from build123d import *

# Parameters (mm, degrees)
F1_DEPTH = 44
F2_R     = 2
F3_DEPTH = 25


with BuildPart() as f1:
    # F0 (on Front) → F1 (new body)
    with BuildSketch(Plane.XZ):
        Polygon((0, 2), (0, 0), (36, 0), (36, 2), (20, 2), (20, 14.713833), (36.245195, 32.134672), (50.505946, 32.134672), (50.505946, 36.134672), (34.505946, 36.134672), (12, 12), (12, 2), align=None)
    extrude(amount=-F1_DEPTH)

    # F2 (on Top) → F3 (cut)
    with BuildSketch(Plane.XY):
        with Locations((4, 40)):
            Circle(F2_R)
        with BuildLine():
            Line((12, 0), (12, 36))
            Line((12, 36), (4, 36))
            ThreePointArc((4, 36), (1.171573, 37.171573), (0, 40))
            Line((0, 40), (0, 0))
            Line((0, 0), (12, 0))
        make_face()
    extrude(amount=F3_DEPTH, mode=Mode.SUBTRACT)


solid = f1.part
The model under review builds one solid part; all positions refer to its coordinate system, in mm. A direction names the side the tool comes from. Round coordinates to 2 decimals unless told otherwise and drop trailing zeros. Loops run counter-clockwise (first coordinate to the right, second up) from the corner with the lowest first, then second, coordinate; pieces in that order, holes last. Notation, with made-up numbers: M 48,-19 L 87,-19 A33 cw 87,17 Z; hole C -1,-39.75 d3. An arc over 180 degrees is marked long. Answer as a JSON object with one key per item and string values.
Item 1: The part is to be moulded in two halves that separate along X. For faces 1 (the face through (1.203, 37.141, 0.986)), 2 (the face through (28, 22, 2)), 3 (the face through (4, 38, 1)), say which applies: +X half, -X half, draft (parallel to the pull), parting line (faces both ways), or undercut.
Check sheet entries:
{"face 1": "-X half", "face 2": "draft", "face 3": "undercut"}
Item 2: We need section C-C, the plane z = 30. State the section outline as (x, y) points, and give its area (3 significant figures).
Check sheet entries:
{"outline": "M 28.79,0 L 34.25,0 L 34.25,44 L 28.79,44 Z", "area": "241 mm2"}
Item 3: We need section B-B, the plane y = 26. State the section outline as (x, z) points.
Check sheet entries:
{"outline": "M 12,0 L 36,0 L 36,2 L 20,2 L 20,14.71 L 36.25,32.13 L 50.51,32.13 L 50.51,36.13 L 34.51,36.13 L 12,12 Z"}
Item 4: We need section A-A, the plane x = 24.5. State the section outline as (y, z) points.
Check sheet entries:
{"outline": "M 0,0 L 44,0 L 44,2 L 0,2 Z; M 0,19.54 L 44,19.54 L 44,25.4 L 0,25.4 Z"}
Item 5: Clearance check with flat-ended pins moving along their axes: P1, Ø1, axis at y = 13.5, z = 22, coming from the +X side; P2, Ø10, axis at y = 30.5, z = 20.5, coming from the -X side; P3, Ø6, axis at x = 26, y = 11.5, coming from the +Z side. State where each tip first meets the part, or that it passes through.
Check sheet entries:
{"P1": "x = 27.26", "P2": "x = 15.26", "P3": "z = 30.23"}
Item 6: For line 1 along X through (y, z) = (40, 1.1); line 2 along Y through (x, z) = (4, 0.6); line 3 along Z through (x, y) = (41, 4.5), list the stretches that pass through material, from the lowest coordinate up.
Check sheet entries:
{"line 1": "0 to 2, 6 to 36", "line 2": "36 to 38, 42 to 44", "line 3": "32.13 to 36.13"}
Item 7: Tool access review of faces 4 (the face through (43, 22, 32.135)), 5 (the face through (8, 36, 1)), 6 (the face through (20, 22, 8)): name each direction out of +Z, -Z, +X, -X, +Y, -Y from which nothing blocks a thin tool from reaching the whole face with its end or side.
Check sheet entries:
{"face 4": "-Z, +X, +Y, -Y", "face 5": "+Z, -Z, -X, -Y", "face 6": "+X, +Y, -Y"}
